Work out the finished part from the listing and answer in its coordinate system (mm). A direction names the side the tool comes from. Give positions to 0.01 mm unless a question says otherwise; leave off trailing zeros. Loops run counter-clockwise (first coordinate to the right, second up) from the corner with the lowest first, then second, coordinate; pieces in that order, holes last. Notation, with made-up numbers: (83, -27.75) -> (103, -27.75) arc R23 cw to (103, -12.75) -> close; hole circle Ø2 at (8.25, -11.5). An arc over 180 degrees is marked (long way). Answer as CSV lines item,"result". Start each with the question number.
1. Find section C-C, the plane x = 9.5. Give the vertices of the cut face in (y, z), and give its area (3 significant figures).
2. A tool of negligible diameter and unlimited length cuts with its end or side. For faces 1 (the face through (16.25, 1.77, 39.06)), 2 (the face through (-36, 2, -45)), from which of +Z, -Z, +X, -X, +Y, -Y can it reach the whole face along a straight path? Write none if from no direction.
3. Find section B-B, the plane y = 0.75. Give the vertices of the cut face in (x, z) (3 decimals).
4. Find section A-A, the plane x = 0. Give the vertices of the cut face in (y, z), and give its area (3 significant figures).
5. Find the intervals of material crossed by line 1 along Z through (x, y) = (-27.5, 2.55) (3 decimals); line 2 along Z through (x, y) = (15.5, 1.25) (3 decimals); line 3 along X through (y, z) = (1.85, 40) (3 decimals), in increasing order.
6. Determine the mould class of faces 3 (the face through (-15, 3.6, -9)), 4 (the face through (16.25, 1.77, -20.94)), 5 (the face through (-52, 2, -1)) for opening direction X: +X half, -X half, draft (parallel to the pull), parting line (faces both ways), or undercut.
7. Flat-ended cylindrical pins translate along their axes: pin 1 Ø2.5 at (x, z) = (-27.5, -40.5) entering from -Y; pin 2 Ø1.8 at (x, y) = (-39.5, 2.5) entering from -Z; pin 3 Ø1.5 at (x, y) = (10, 0.5) entering from -Z. Find the tip coordinate at first contact, or state that the pin passes through.
Autodesk Inventor part; units mm, degrees
ref_plane "YZ Plane" through (0, 0, 0) normal (1, 0, 0) x (0, 1, 0)
ref_plane "XZ Plane" through (0, 0, 0) normal (0, 1, 0) x (-1, 0, 0)
ref_plane "XY Plane" through (0, 0, 0) normal (0, 0, 1) x (1, 0, 0)
sketch "Sketch1" plane through (0, 0, 0) normal (0, 1, 0) x (-1, 0, 0)
  line L0 (20, 45) -> (-20, 45)
  line L1 (-20, 45) -> (-20, -45)
  line L2 (-20, -45) -> (20, -45)
  line L3 (20, -45) -> (20, 45)
  line L4 (20, 45) -> (-20, -45) construction
  line L5 (-20, 45) -> (20, -45) construction
  arc A0 (-20, -45) -> (20, -45) centre (0, -45) ccw
  line L6 (20, -45) -> (52, -45)
  line L7 (52, -45) -> (52, 45)
  line L8 (52, 45) -> (20, 45)
  line L9 (20, 45) -> (20, -45)
  point P0 (0, 0)
  dimension "d0" = 40
  dimension "d1" = 90
  dimension "d7" = 32
  dimension "d8" = 90
extrude "Extrusion1" add sketch "Sketch1" along normal blind 3.6
sketch "Sketch2" plane through (0, 3.6, 0) normal (0, 1, 0) x (1, 0, 0)
  arc A0 (20, 45) -> (-20, 45) centre (0, 45) ccw
  circle A1 centre (0, 45) radius 5.15
  point P0 (0, 0)
  dimension "d4" = 10.3
extrude "Extrusion2" cut sketch "Sketch2" against normal blind 3.6
fillet "Fillet1" radius 4 4 edges at (-20, 1.8, -45) (-52, 1.8, -45) (-52, 1.8, 45) (20, 1.8, 45)
sketch "Sketch3" plane through (0, 0, 0) normal (0, -1, 0) x (1, 0, 0)
  circle A0 centre (15.5, 40.5) radius 1.625
  circle A1 centre (15.5, -19.5) radius 1.625
  circle A2 centre (-27.5, -40.5) radius 1.625
  line L0 (-52, -41) -> (-52, 41)
  line L1 (-23.6643, -45) -> (-48, -45)
  line L2 (20, 41) -> (20, -45)
  line L3 (-48, 45) -> (16, 45)
  point P0 (0, 0)
  dimension "d10" = 3.25
  dimension "d11" = 3.25
  dimension "d12" = 3.25
  dimension "d13" = 24.5
  dimension "d14" = 4.5
  dimension "d15" = 4.5
  dimension "d16" = 4.5
  dimension "d17" = 4.5
  dimension "d18" = 60
extrude "Extrusion3" cut sketch "Sketch3" against normal blind 3.8
sketch "Sketch4" plane through (0, 3.6, 0) normal (0, 1, 0) x (1, 0, 0)
  circle A0 centre (-48, -40) radius 1.575
  line L0 (-48, -45) -> (16, -45)
  line L1 (-52, 41) -> (-52, -41)
  point P0 (0, 0)
  dimension "d21" = 3.15
  dimension "d22" = 5
  dimension "d23" = 4
extrude "Extrusion4" cut sketch "Sketch4" against normal blind 3.8
properties part number "p1"
Resolved:
1,outline,"(0, -62.6) -> (3.6, -62.6) -> (3.6, 45) -> (0, 45) -> close"
1,area,"387 mm^2"
2,face 1,"+Y, -Y"
2,face 2,"-Z, -X, +Y, -Y"
3,outline,"(-52, -41) arc R4 ccw to (-48, -45) -> (-23.664, -45) arc R4 cw to (-19.72, -48.333) arc R20 ccw to (20, -45) -> (20, 41) arc R4 ccw to (16, 45) -> (-48, 45) arc R4 ccw to (-52, 41) -> close; hole circle Ø3.15 at (-48, 40); hole circle Ø3.25 at (-27.5, -40.5); hole circle Ø10.3 at (0, -45); hole circle Ø3.25 at (15.5, -19.5); hole circle Ø3.25 at (15.5, 40.5)"
4,outline,"(0, -65) -> (3.6, -65) -> (3.6, -50.15) -> (0, -50.15) -> close; (0, -39.85) -> (3.6, -39.85) -> (3.6, 45) -> (0, 45) -> close"
4,area,"359 mm^2"
5,line 1,"z = -45 to -42.125, -38.875 to 45"
5,line 2,"z = -57.639 to -21.125, -17.875 to 38.875, 42.125 to 45"
5,line 3,"x = -52 to -49.575, -46.425 to 13.954, 17.046 to 20"
6,face 3,"draft"
6,face 4,"undercut"
6,face 5,"-X half"
7,pin 1,"passes through"
7,pin 2,"stops at z = -45"
7,pin 3,"stops at z = -62.73"
